The model under review builds one solid part; all positions refer to its coordinate system, in mm. A direction names the side the tool comes from. Round coordinates to 2 decimals unless told otherwise and drop trailing zeros. Loops run counter-clockwise (first coordinate to the right, second up) from the corner with the lowest first, then second, coordinate; pieces in that order, holes last. Notation, with made-up numbers: (-12.75, 68) -> (7.25, 68) arc R25 ccw to (7.25, 83) -> close; hole circle Ø6 at (-26, 50). An arc over 180 degrees is marked (long way). Use a Markdown table: item, result. Add a question column.
1) Consider section B-B on z = 5.25. Give the boundary of the cut face in (x, y).
2) Insertion check: pin 1 (6 mm diameter, centred on x = -14, z = 5, fed in from +Y); pin 2 (4 mm diameter, centred on y = -13.5, z = 7.5, fed in from +X); pin 3 (13.5 mm diameter, centred on x = 6.5, y = 0.5, fed in from +Z); pin 4 (8 mm diameter, centred on x = -6, y = -16.5, fed in from +Z). Each pin has a flat end and moves straight along its axis. Give the tip position at first contact, or say it passes through.
3) Wall thickness on probe 1 along Y at (x, z) = (0, 1.75); probe 2 along Y at (x, z) = (0, 4.25); probe 3 along Z at (x, y) = (21, -7): over which ranges is each line inside the solid? List them lowest first.
4) Mouldability with a two-part tool opening along X and no side actions: class faces 1 (the flat face through (-10.32, -9.69, 4)), 2 (the cylindrical face through (-5.961, -26.846, 4.93)), 3 (the flat face through (-13, 6, 0)), 4 (the cylindrical face through (-22.65, -12.46, 4.93)) as released by +X, released by -X, zero draft, split by the parting line, or undercut.
5) For faces 5 (the cylindrical face through (0, 24, 5)), 6 (the cylindrical face through (10.382, -19.961, 6.958)), list the 3-axis set-ups (+Z, -Z, +X, -X, +Y, -Y) from which the entire face can be reached by the end or side of a thin tool; tool diameter is ignored.
6) Consider section D-D on x = 7.5. Give the boundary of the cut face in (y, z).
7) Consider section C-C on y = -12.5. Give the boundary of the cut face in (x, z).
8) Consider section A-A on y = 0. Give the boundary of the cut face in (x, z).
from build123d import *

# Parameters (mm, degrees)
SKETCH_R      = 27.5
SKETCH_R_2    = 22.5
SKETCH_R_3    = 1
PAD_DEPTH     = 10
SKETCH001_R   = 22.5
SKETCH001_R_2 = 14
PAD001_DEPTH  = 4


with BuildPart() as part:
    # Sketch → Pad (new body)
    with BuildSketch(Plane.XY):
        Circle(SKETCH_R)
        Circle(SKETCH_R_2, mode=Mode.SUBTRACT)
        with Locations((0, 25)):
            Circle(SKETCH_R_3, mode=Mode.SUBTRACT)
        with Locations((-21.650635, -12.5)):
            Circle(SKETCH_R_3, mode=Mode.SUBTRACT)
        with Locations((21.650635, -12.5)):
            Circle(SKETCH_R_3, mode=Mode.SUBTRACT)
    extrude(amount=PAD_DEPTH)

    # Sketch001 → Pad001 (join)
    with BuildSketch(Plane.XY):
        Circle(SKETCH001_R)
        Circle(SKETCH001_R_2, mode=Mode.SUBTRACT)
    extrude(amount=PAD001_DEPTH)


solid = part.part
Result set:
| question | item | result |
|---|---|---|
| 1 | outline | circle Ø55 at (0, 0); hole circle Ø2 at (-21.65, -12.5); hole circle Ø45 at (0, 0); hole circle Ø2 at (0, 25); hole circle Ø2 at (21.65, -12.5) |
| 2 | pin 1 | y = 25.2 |
| 2 | pin 2 | x = 24.98 |
| 2 | pin 3 | through |
| 2 | pin 4 | z = 4 |
| 3 | probe 1 | -27.5 to -14, 14 to 24, 26 to 27.5 |
| 3 | probe 2 | -27.5 to -22.5, 22.5 to 24, 26 to 27.5 |
| 3 | probe 3 | 0 to 4 |
| 4 | face 1 | undercut |
| 4 | face 2 | split by the parting line |
| 4 | face 3 | zero draft |
| 4 | face 4 | undercut |
| 5 | face 5 | +Z, -Z |
| 5 | face 6 | +Z |
| 6 | outline | (-26.46, 0) -> (-11.82, 0) -> (-11.82, 4) -> (-21.21, 4) -> (-21.21, 10) -> (-26.46, 10) -> close; (11.82, 0) -> (26.46, 0) -> (26.46, 10) -> (21.21, 10) -> (21.21, 4) -> (11.82, 4) -> close |
| 7 | outline | (-24.49, 0) -> (-22.65, 0) -> (-22.65, 10) -> (-24.49, 10) -> close; (-20.65, 0) -> (-6.3, 0) -> (-6.3, 4) -> (-18.71, 4) -> (-18.71, 10) -> (-20.65, 10) -> close; (6.3, 0) -> (20.65, 0) -> (20.65, 10) -> (18.71, 10) -> (18.71, 4) -> (6.3, 4) -> close; (22.65, 0) -> (24.49, 0) -> (24.49, 10) -> (22.65, 10) -> close |
| 8 | outline | (-27.5, 0) -> (-14, 0) -> (-14, 4) -> (-22.5, 4) -> (-22.5, 10) -> (-27.5, 10) -> close; (14, 0) -> (27.5, 0) -> (27.5, 10) -> (22.5, 10) -> (22.5, 4) -> (14, 4) -> close |
